Design review of the part shown in the three views and the two pictorial views. Dimensions are in mm from the part's minimum x, y and z. Coordinates: 2 decimals unless noted, no trailing zeros. Loops run counter-clockwise (first coordinate to the right, second up) from the corner with the lowest first, then second, coordinate; pieces in that order, holes last. Notation, with made-up numbers: (-39.75, -10) -> (18.25, -10) arc R24 cw to (18.25, 16) -> close; hole circle Ø2 at (50, 35). An arc over 180 degrees is marked (long way). Use a Markdown table: item, result. Add a question column.
Q1. Take a section at C-C on x = 90. Write out the cut boundary in (y, z).
Q2. Take a section at A-A on y = 5. Write out the cut boundary in (x, z), plus the area to 3 significant figures.
Q3. For probe 1 along X at (y, z) = (5.25, 6.5); probe 2 along Y at (x, z) = (90, 7); probe 3 along Y at (x, z) = (3, 2), list the stretches that pass through material, from the lowest coordinate up.
Q4. Take a section at D-D on y = 9. Write out the cut boundary in (x, z).
Q5. Clearance check with flat-ended pins moving along their axes: pin 1 Ø2.5 at (x, y) = (3, 5) entering from +Z; pin 2 Ø1.5 at (x, z) = (77, 2.5) entering from -Y; pin 3 Ø4 at (x, y) = (34.5, 9) entering from +Z; pin 4 Ø1.5 at (x, y) = (77, 6.5) entering from +Z. State where each tip first meets the part, or that it passes through.
Q6. Take a section at B-B on z = 5. Write out the cut boundary in (x, y), plus the area to 3 significant figures.
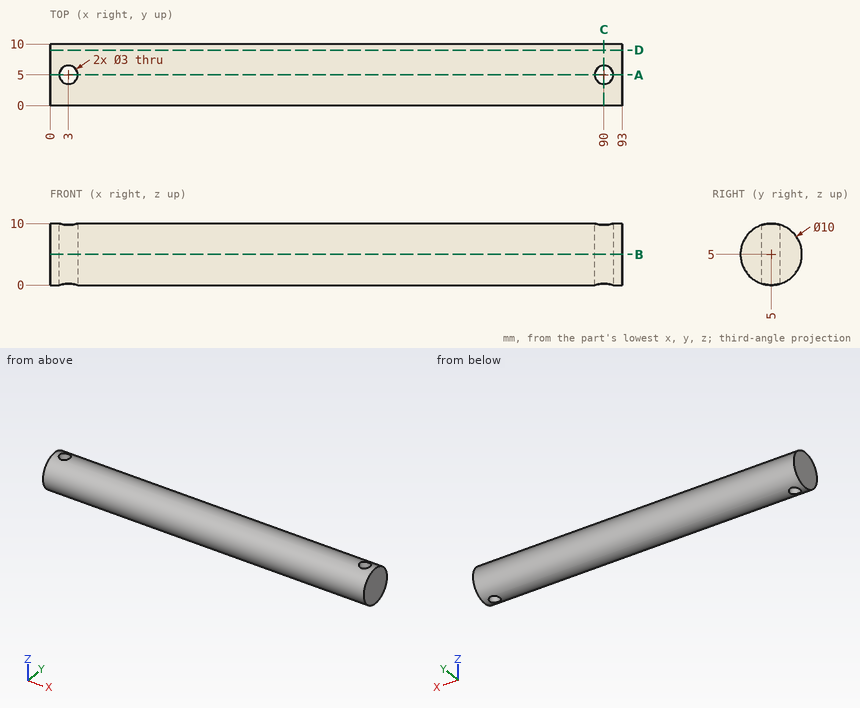
Answer list:
| question | item | result |
|---|---|---|
| 1 | outline | (3.5, 0.23) -> (3.5, 9.77) arc R5 ccw to start; (6.5, 0.23) arc R5 ccw to (6.5, 9.77) -> close |
| 2 | outline | (0, 0) -> (1.5, 0) -> (1.5, 10) -> (0, 10) -> close; (4.5, 0) -> (88.5, 0) -> (88.5, 10) -> (4.5, 10) -> close; (91.5, 0) -> (93, 0) -> (93, 10) -> (91.5, 10) -> close |
| 2 | area | 870 mm² |
| 3 | probe 1 | 0 to 1.52, 4.48 to 88.52, 91.48 to 93 |
| 3 | probe 2 | 0.42 to 3.5, 6.5 to 9.58 |
| 3 | probe 3 | 1 to 3.5, 6.5 to 9 |
| 4 | outline | (0, 2) -> (93, 2) -> (93, 8) -> (0, 8) -> close |
| 5 | pin 1 | through |
| 5 | pin 2 | y = 0.32 |
| 5 | pin 3 | z = 9.58 |
| 5 | pin 4 | z = 9.94 |
| 6 | outline | (0, 0) -> (93, 0) -> (93, 10) -> (0, 10) -> close; hole circle Ø3 at (3, 5); hole circle Ø3 at (90, 5) |
| 6 | area | 916 mm² |
